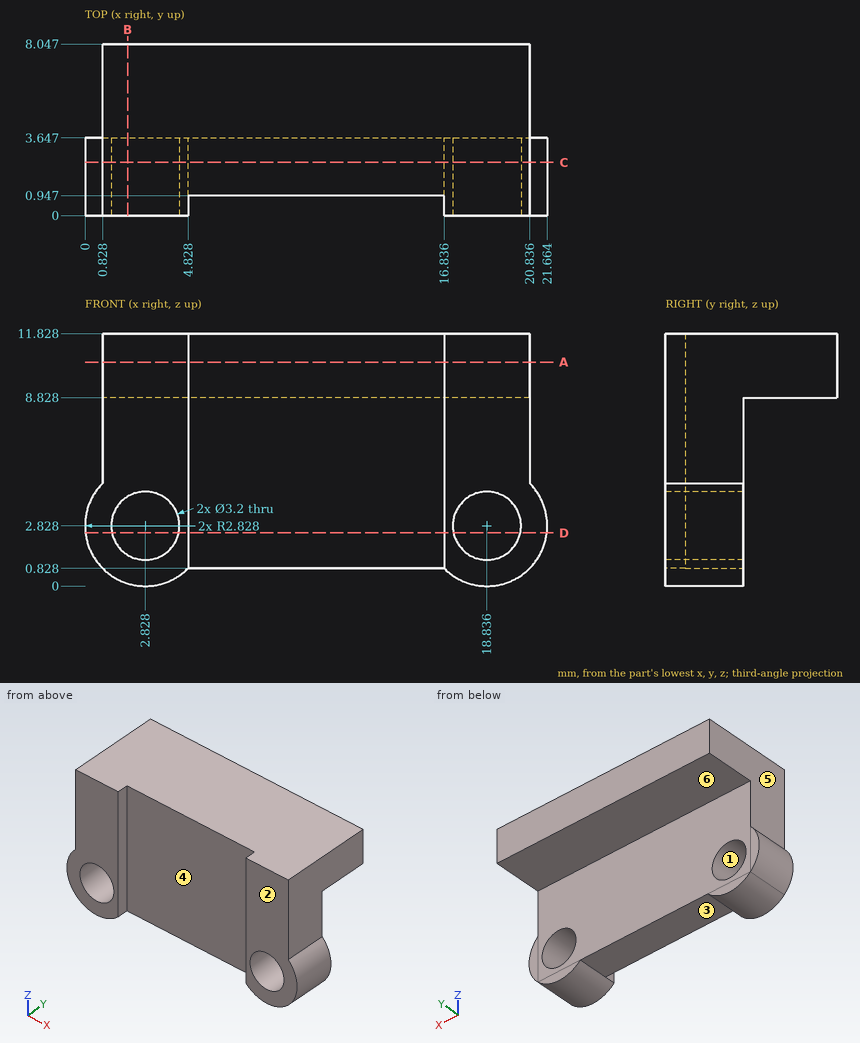
Design review of the part shown in the three views and the two pictorial views. Dimensions are in mm from the part's minimum x, y and z. A direction names the side the tool comes from. Round coordinates to 2 decimals unless told otherwise and drop trailing zeros. Loops run counter-clockwise (first coordinate to the right, second up) from the corner with the lowest first, then second, coordinate; pieces in that order, holes last. Notation, with made-up numbers: (82, 89.25) - (133, 89.25) arc R30 ccw to (133, 125.25) - close; hole circle Ø1 at (-29, 26). An arc over 180 degrees is marked (long way). Answer as CSV lines item,"result".
(1) Tool access review of the marked faces 4, 5 and 6: name each direction out of +Z, -Z, +X, -X, +Y, -Y from which nothing blocks a thin tool from reaching the whole face with its end or side.
Checked values:
face 4,"+Z, -Z, -Y"
face 5,"+Z, -X, +Y, -Y"
face 6,"-Z, +X, -X, +Y"
(2) Mouldability with a two-part tool opening along Z and no side actions: class the marked faces 1, 2 and 3 as +Z half, -Z half, draft (parallel to the pull), parting line (faces both ways), or undercut.
Checked values:
face 1,"undercut"
face 2,"draft"
face 3,"-Z half"
(3) Consider section C-C on y = 2.5. Give the boundary of the cut face in (x, z), then the cut area to 3 significant figures.
Checked values:
outline,"(0.83, 4.83) arc R2.83 ccw to (4.83, 0.83) - (16.84, 0.83) arc R2.83 ccw to (20.84, 4.83) - (20.84, 11.83) - (0.83, 11.83) - close; hole circle Ø3.2 at (2.83, 2.83); hole circle Ø3.2 at (18.84, 2.83)"
area,"213 mm2"
(4) Insertion check: P1, Ø4, axis at x = 11.5, y = 2, coming from the -Z side; P2, Ø4, axis at x = 12.5, y = 7, coming from the -Z side; P3, Ø0.7, axis at x = 18.5, z = 0.5, coming from the +Y side; P4, Ø1.9, axis at x = 2.83, z = 2.83, coming from the +Y side. Each pin has a flat end and moves straight along its axis. Give the tip position at first contact, or say it passes through.
Checked values:
P1,"stops at z = 0.83"
P2,"stops at z = 8.83"
P3,"stops at y = 3.65"
P4,"passes through"
(5) Consider section B-B on x = 2. Give the boundary of the cut face in (y, z), then the cut area to 3 significant figures.
Checked values:
outline,"(0, 0.12) - (3.65, 0.12) - (3.65, 1.46) - (0, 1.46) - close; (0, 4.2) - (3.65, 4.2) - (3.65, 8.83) - (8.05, 8.83) - (8.05, 11.83) - (0, 11.83) - close"
area,"45.9 mm2"
(6) Consider section A-A on z = 10.5. Give the boundary of the cut face in (x, y), then the cut area to 3 significant figures.
Checked values:
outline,"(0.83, 0) - (4.83, 0) - (4.83, 0.95) - (16.84, 0.95) - (16.84, 0) - (20.84, 0) - (20.84, 8.05) - (0.83, 8.05) - close"
area,"150 mm2"
(7) Wall thickness on line 1 (Y direction, x = 8.5, z = 6.5); line 2 (Y direction, x = 19.25, z = 5); line 3 (Z direction, x = 20, y = 7.5): over which ranges is each line inside the solid? List them lowest first.
Checked values:
line 1,"y = 0.95 to 3.65"
line 2,"y = 0 to 3.65"
line 3,"z = 8.83 to 11.83"
(8) Consider section D-D on z = 2.5. Give the boundary of the cut face in (x, y) (1 decimal).
Checked values:
outline,"(0, 0) - (1.3, 0) - (1.3, 3.6) - (0, 3.6) - close; (4.4, 0) - (4.8, 0) - (4.8, 0.9) - (16.8, 0.9) - (16.8, 0) - (17.3, 0) - (17.3, 3.6) - (4.4, 3.6) - close; (20.4, 0) - (21.6, 0) - (21.6, 3.6) - (20.4, 3.6) - close"
